CAD build for the part. Positions are in the model's coordinates, mm. A direction names the side the tool comes from. Round coordinates to 2 decimals unless told otherwise and drop trailing zeros. Loops run counter-clockwise (first coordinate to the right, second up) from the corner with the lowest first, then second, coordinate; pieces in that order, holes last. Notation, with made-up numbers: M 45,51.5 L 99,51.5 A26 ccw 99,76.5 Z; hole C -18,-5.75 d3. An arc over 180 degrees is marked long. Use one line per item in the form item = value.
from build123d import *

# Parameters (mm, degrees)
F0_W     = 70
F0_H     = 33
F0_R     = 1.4
F1_DEPTH = 43.3
F3_DEPTH = 40
F4_W     = 53
F4_H     = 6
F5_DEPTH = 7
F6_W     = 53
F6_H     = 6
F7_DEPTH = 7


with BuildPart() as f1:
    # F0 (on Top) → F1 (new body)
    with BuildSketch(Plane.XY):
        Rectangle(F0_W, F0_H)
        Circle(F0_R, mode=Mode.SUBTRACT)
    extrude(amount=F1_DEPTH)

    # F2 (on face) → F3 (cut)
    with BuildSketch(Plane(origin=(0, 0, 0), x_dir=(1, 0, 0), z_dir=(0, 0, -1))):
        with BuildLine():
            Line((4, 18.442246), (-4, 18.442246))
            Line((-4, 18.442246), (-4, 0))
            ThreePointArc((-4, 0), (0, -4), (4, 0))
            Line((4, 0), (4, 18.442246))
        make_face()
    extrude(amount=-F3_DEPTH, mode=Mode.SUBTRACT)

    # F4 (on face) → F5 (cut)
    with BuildSketch(Plane.XZ.offset(16.5)):
        with Locations((0, 4.5)):
            Rectangle(F4_W, F4_H)
    extrude(amount=-F5_DEPTH, mode=Mode.SUBTRACT)

    # F6 (on face) → F7 (cut)
    with BuildSketch(Plane(origin=(0, 16.5, 0), x_dir=(-1, 0, 0), z_dir=(0, 1, 0))):
        with Locations((0, 4.5)):
            Rectangle(F6_W, F6_H)
    extrude(amount=-F7_DEPTH, mode=Mode.SUBTRACT)


solid = f1.part
1. Probe line 1 along X through (y, z) = (0, 41.7); line 2 along X through (y, z) = (-14, 8.5); line 3 along Y through (x, z) = (0, 40.7). List the from-to ranges inside material, lowest first. Write a range as from..to.
Completed:
line_1 = -35..-1.4, 1.4..35
line_2 = -35..-4, 4..35
line_3 = -16.5..-1.4, 1.4..16.5
2. Cut at D-D on x = 15.5. Write the cut outline in (y, z), and give its area (3 significant figures).
Completed:
outline = M -16.5,0 L 16.5,0 L 16.5,1.5 L 9.5,1.5 L 9.5,7.5 L 16.5,7.5 L 16.5,43.3 L -16.5,43.3 L -16.5,7.5 L -9.5,7.5 L -9.5,1.5 L -16.5,1.5 Z
area = 1,340 mm2
3. Cut at C-C on y = -4. Write the cut outline in (x, z), and give its area (3 significant figures).
Completed:
outline = M -35,0 L -4,0 L -4,40 L 4,40 L 4,0 L 35,0 L 35,43.3 L -35,43.3 Z
area = 2,710 mm2
4. Drop flat-ended pins along their axis: P1, Ø1.8, axis at x = -12.5, z = 5.5, coming from the -Y side; P2, Ø1.8, axis at x = -9, z = 5.5, coming from the +Y side; P3, Ø4, axis at x = 1, y = -8, coming from the -Z side. Give the stop position or say it passes through.
Completed:
P1 = -9.5
P2 = 9.5
P3 = 40
5. Cut at A-A on x = 0. Write the cut outline in (y, z), and give its area (3 significant figures).
Completed:
outline = M -16.5,40 L -1.4,40 L -1.4,43.3 L -16.5,43.3 Z; M 1.4,40 L 4,40 L 4,0 L 16.5,0 L 16.5,1.5 L 9.5,1.5 L 9.5,7.5 L 16.5,7.5 L 16.5,43.3 L 1.4,43.3 Z
area = 558 mm2
6. Cut at B-B on z = 36.5. Write the cut outline in (x, y), and give its area (3 significant figures).
Completed:
outline = M -35,-16.5 L -4,-16.5 L -4,0 A4 cw 4,0 L 4,-16.5 L 35,-16.5 L 35,16.5 L -35,16.5 Z
area = 2,150 mm2
7. Pull direction Z, two halves, no side cores. Call faces 1 (the face through (-26.5, 13, 4)), 2 (the face through (0, 4, 43.3)), 3 (the face through (0, 4, 20)): +Z half, -Z half, draft (parallel to the pull), parting line (faces both ways), or undercut.
Completed:
face_1 = undercut
face_2 = +Z half
face_3 = draft
8. Tool access for faces 4 (the face through (26.5, -13, 4)), 5 (the face through (0, 13, 1.5)), 6 (the face through (0, -6, 40)): list every direction of +Z, -Z, +X, -X, +Y, -Y with a clear straight run to the whole face (end or side of a thin tool).
Completed:
face_4 = -Y
face_5 = +Y
face_6 = -Z, -Y
